Autodesk Inventor part; units mm, degrees
ref_plane "YZ Plane" through (0, 0, 0) normal (1, 0, 0) x (0, 1, 0)
ref_plane "XZ Plane" through (0, 0, 0) normal (0, 1, 0) x (-1, 0, 0)
ref_plane "XY Plane" through (0, 0, 0) normal (0, 0, 1) x (1, 0, 0)
sketch "Эскиз1" plane through (0, 0, 0) normal (0, 0, 1) x (1, 0, 0)
  line L0 (0, 0) -> (-52, 0)
  line L1 (-52, 0) -> (-52, -28) construction
  line L2 (-52, -28) -> (0, -28)
  line L3 (0, -28) -> (0, 0)
  arc A0 (-52, 0) -> (-52, -28) centre (-52, -14) ccw
  point P0 (-66, -14)
  dimension "d1" = 28
  dimension "d2" = 66
extrude "Выдавливание1" add sketch "Эскиз1" along normal blind 26.5
fillet "Сопряжение1" radius 2 2 edges at (0, -14, 26.5) (0, -14, 0)
fillet "Сопряжение2" radius 2 12 edges at (-0.5858, 0, 25.9142) (-27, 0, 26.5) (-66, -14, 26.5) (-27, -28, 26.5) (-0.5858, -28, 25.9142) (0, -28, 13.25) (-0.5858, -28, 0.5858) (-27, -28, 0) (-66, -14, 0) (-27, 0, 0) (-0.5858, 0, 0.5858) (0, 0, 13.25)
sketch "Эскиз2" plane through (0, -26, 24.5) normal (1, 0, 0) x (0, 0, -1)
  line L0 (6.0366, 15.0348) -> (16.61, 15.0348)
  line L1 (16.61, 15.0348) -> (16.61, 8.9331)
  line L2 (16.61, 8.9331) -> (6.0366, 8.9331)
  line L3 (6.0366, 8.9331) -> (6.0366, 15.0348)
  point P0 (24.5, 26)
extrude "Выдавливание2" add sketch "Эскиз2" against normal blind 95
properties part number "bat_sketch"
Input: part model. Units: mm. Frame: model coordinates. A direction names the side the tool comes from. Give positions to 0.01 mm unless a question says otherwise; leave off trailing zeros. Loops run counter-clockwise (first coordinate to the right, second up) from the corner with the lowest first, then second, coordinate; pieces in that order, holes last. Notation, with made-up numbers: M -29.5,13 L 3.5,13 A15 cw 3.5,34 Z; hole C 31.5,-18 d9. An arc over 180 degrees is marked long. Answer as CSV lines item,"result". Start each with the question number.
1. Section A-A on y = -14. Return loops of the section in (x, z).
2. Reachability of faces 1 (the face through (-80, -10.965, 13)), 2 (the face through (-0.57, -0.6, 13.41)), 3 (the face through (-80, -17.067, 13)) from +Z, -Z, +X, -X, +Y, -Y: full face, straight path, thin tool, end or side. Return the list, or none.
3. Section B-B on z = 19.5. Return loops of the section in (x, y).
4. Pin query (flat end, axial travel): P1, Ø8, axis at y = -20.5, z = 19, coming from the -X side; P2, Ø3, axis at x = -74.5, y = -15, coming from the +Z side; P3, Ø8.5, axis at x = -84, z = 11.5, coming from the +Y side; P4, Ø3, axis at x = -78, y = -15, coming from the -Z side. Return the tip coordinate at first contact, or that it passes through.
5. Section C-C on x = -79. Return loops of the section in (y, z), plus the area to 3 significant figures.
6. Line query: L1, parallel to Z at x = -79, y = -14; L2, parallel to X at y = -14, z = 2.5; L3, parallel to Y at x = -70, z = 14.5. Output: solid intervals per line, ascending.
Computed values:
1,outline,"M -95,7.89 L -66,7.89 L -66,2 A2 ccw -64,0 L -2,0 A2 ccw 0,2 L 0,24.5 A2 ccw -2,26.5 L -64,26.5 A2 ccw -66,24.5 L -66,18.46 L -95,18.46 Z"
2,face 1,"+Z, -Z, -X, +Y"
2,face 2,"+Z, -Z, +X, +Y"
2,face 3,"+Z, -Z, -X, -Y"
3,outline,"M -52,-28 L -2,-28 A2 ccw 0,-26 L 0,-2 A2 ccw -2,0 L -52,0 A14 ccw Z"
4,P1,"stops at x = -95"
4,P2,"stops at z = 18.46"
4,P3,"stops at y = -10.97"
4,P4,"stops at z = 7.89"
5,outline,"M -17.07,7.89 L -10.97,7.89 L -10.97,18.46 L -17.07,18.46 Z"
5,area,"64.5 mm²"
6,L1,"z = 7.89 to 18.46"
6,L2,"x = -66 to 0"
6,L3,"y = -17.07 to -10.97"
